CAD build for the part. Positions are in the model's coordinates, mm. A direction names the side the tool comes from. Coordinates: 2 decimals unless noted, no trailing zeros. Order: outer loops, then holes, each group sorted by start corner. A loop starts at its lowest first (then second) coordinate and runs counter-clockwise, first axis right, second up. Notation, with made-up numbers: M 19.25,87 L 30.25,87 A24 ccw 30.25,112 Z; hole C 10.25,2 d5. An arc over 180 degrees is marked long. One line per item, written item: value.
from build123d import *

# Parameters (mm, degrees)
ESQUISSE2_R                  = 30
ESQUISSE2_R_2                = 11
ENL_V_MAT_EXTRU_2_DEPTH      = 10
ESQUISSE4_R                  = 4
ENL_V_MAT_EXTRU_3_DEPTH      = 65.601563534
ESQUISSE5_R                  = 6
ENL_V_MAT_EXTRU_4_DEPTH      = 65.601563534
R_P_TITION_CIRCULAIRE1_COUNT = 2
R_P_TITION_CIRCULAIRE1_ANGLE = 180


with BuildPart() as part:
    # Esquisse1 → Révolution1 (revolve)
    with BuildSketch(Plane.XY, mode=Mode.PRIVATE) as r_volution1_sk:
        Polygon((-0.603091605, -37), (-1.414213562, -37), (0, -35.585786438), (0, -4.5), (-20.414163341, -4.5), (-23.429029468, -7.514866127), (-43.429029468, -7.514866127), (-44.957951939, -8.804205522), (-44.957951939, -11), (-36.957951939, -11), (-36.957951939, -11.014343795), (-34.957951939, -11.014343795), (-34.957951939, -15.337655327), (-34.957951939, -27.510373989), (-34.957951939, -32.507595335), (-15.957951939, -32.507595335), (-15.957951939, -36.740873266), (-14.862537746, -38.414213562), (-2.017305168, -38.414213562), align=None)
    revolve(r_volution1_sk.sketch.rotate(Axis((0, 0, 0), (-1, 0, 0)), 180), axis=Axis((0, 0, 0), (-1, 0, 0)))

    # Esquisse2 → Enlèv. mat.-Extru.2 (cut)
    with BuildSketch(Plane(origin=(0, 0, 0), x_dir=(0, 0, -1), z_dir=(1, 0, 0))):
        Circle(ESQUISSE2_R)
        with Locations(Location((0, 0, 0), (0, 0, 90))):
            Circle(ESQUISSE2_R_2, mode=Mode.SUBTRACT)
    extrude(amount=-ENL_V_MAT_EXTRU_2_DEPTH, mode=Mode.SUBTRACT)

    # Esquisse4 → Enlèv. mat.-Extru.3 (cut, through all)
    with BuildSketch(Plane(origin=(-10, 0, 0), x_dir=(0, 0, -1), z_dir=(1, 0, 0))):
        with Locations((21, 0)):
            Circle(ESQUISSE4_R)
        with Locations(Location((-21, 0, 0), (0, 0, 90))):
            Circle(ESQUISSE4_R)
    extrude(amount=-ENL_V_MAT_EXTRU_3_DEPTH, mode=Mode.SUBTRACT)

    # Esquisse5 → Enlèv. mat.-Extru.4 (cut, through all)
    with BuildSketch(Plane(origin=(-10, 0, 0), x_dir=(0, 0, -1), z_dir=(1, 0, 0))):
        with Locations((0, 21)):
            Circle(ESQUISSE5_R)
    enl_v_mat_extru_4 = extrude(amount=-ENL_V_MAT_EXTRU_4_DEPTH, mode=Mode.SUBTRACT)

    # Répétition circulaire1: Enlèv. mat.-Extru.4 ×2 about axis
    r_p_tition_circulaire1_axis = Axis((0, 0, 0), (1, 0, 0))
    for i in range(1, R_P_TITION_CIRCULAIRE1_COUNT):
        add(enl_v_mat_extru_4.rotate(r_p_tition_circulaire1_axis, i * R_P_TITION_CIRCULAIRE1_ANGLE / (R_P_TITION_CIRCULAIRE1_COUNT - 1)), mode=Mode.SUBTRACT)


solid = part.part
Q1. Slice it at D-D (x = -29). List the corners of the cut face in (y, z).
Recorded:
outline: C 0,0 d65.02; hole C -21,0 d12; hole C 0,0 d15.03; hole C 0,-21 d8; hole C 0,21 d8; hole C 21,0 d12
Q2. Mould opens along Y. For faces 3 (the face through (-34.958, -14, 0)), 4 (the face through (-33.569, -7.508, -0.33)), 5 (the face through (-10, 0, -13)), 6 (the face through (-25.325, -7.047, 31.735)) say: released by +Y, released by -Y, zero draft, split by the parting line, or undercut.
Recorded:
face 3: zero draft
face 4: undercut
face 5: undercut
face 6: split by the parting line
Q3. Slice it at A-A (y = 0). Give the number of separate pieces and of enclosed holes in the cut face, plus the area to 3 significant figures.
Recorded:
separate pieces: 4
enclosed holes: 0
area: 1,350 mm^2
Q4. Which spindle directions (+Z, -Z, +X, -X, +Y, -Y) get a long thin tool onto all of the face, cutting with end or side? Do faces 1 (the face through (-40.9, -2.38, 10.74)), 2 (the face through (-22, -21, -6)). Say none if no direction does.
Recorded:
face 1: -X
face 2: +X, -X
Q5. Slice it at B-B (x = -6.5). List the corners of the cut face in (y, z), plus the area to 3 significant figures.
Recorded:
outline: C 0,0 d76.83; C 0,0 d22; hole C 0,0 d60; hole C 0,0 d9
area: 2,120 mm^2
Q6. Pin check, flat tips, straight feed: pin 1 Ø7 at (y, z) = (-21, 0) entering from +X; pin 2 Ø5 at (x, z) = (-29, -12.5) entering from +Y; pin 3 Ø12 at (y, z) = (21, 6) entering from -X; pin 4 Ø6 at (x, y) = (-36.5, 10) entering from -Z. Stop position of each tip, or through.
Recorded:
pin 1: passes through
pin 2: stops at y = 30.93
pin 3: stops at x = -34.96
pin 4: stops at z = -31.65
Q7. Drill centre lines: line 1 along Z through (x, y) = (-27, -3); line 2 along X through (y, z) = (9.5, 28.5); line 3 along X through (y, z) = (6, 22.5). Where is each one in solid material? Low to high.
Recorded:
line 1: z = -32.37 to -23.65, -18.35 to -6.89, 6.89 to 18.35, 23.65 to 32.37
line 2: x = -34.96 to 0
line 3: x = -34.96 to -10
